Build history of the part. All positions in model axes, mm. Round coordinates to 2 decimals unless told otherwise and drop trailing zeros. One line per item, written item: value. Start each with the question number.
Item 1: Pin check, flat tip, straight feed: pin 1 (4 mm diameter, centred on x = 0, y = 0, fed in from +Z). Stop position of the tip, or through.
Item 2: Probe L1, parallel to X at y = 0, z = 8.5; L2, parallel to Y at x = -1, z = 9. List the from-to ranges inside material, lowest first.
Item 3: Two-plate mould, pull along X, no slides. Class faces 1 (the flat face through (11.5, 0, 11)), 2 (the flat face through (0, -11.5, 11)), 3 (the cylindrical face through (-0.195, 1.487, 11.579)): +X half, -X half, draft (parallel to the pull), parting line (faces both ways), or undercut.
```python
from build123d import *

# Parameters (mm, degrees)
SKETCH_W        = 23
SKETCH_H        = 23
PAD_DEPTH       = 23
SKETCH001_R     = 1.5
POCKET_DEPTH    = 23.001
CHAMFER_1_ANGLE = 60
CHAMFER_1_SIZE  = 2.75
CHAMFER_2_ANGLE = 60
CHAMFER_2_SIZE  = 2.75
FILLET_R        = 4


with BuildPart() as part:
    # Sketch → Pad (new body)
    with BuildSketch(Plane.XY):
        Rectangle(SKETCH_W, SKETCH_H)
    extrude(amount=PAD_DEPTH)

    # Sketch001 (on Face6 of Pad) → Pocket (cut, through all)
    with BuildSketch(Plane.XY.offset(23)):
        Circle(SKETCH001_R)
    extrude(amount=-POCKET_DEPTH, mode=Mode.SUBTRACT)

    # Chamfer 1
    chamfer_1_edges = [part.edges().sort_by_distance(p)[0] for p in [
        (-1.5, 0, 23),
    ]]
    chamfer_1_side = part.faces().sort_by_distance((-11.174731, 0, 23))[0]
    chamfer(chamfer_1_edges, length=CHAMFER_1_SIZE, angle=CHAMFER_1_ANGLE, reference=chamfer_1_side)

    # Chamfer 2
    chamfer_2_edges = [part.edges().sort_by_distance(p)[0] for p in [
        (-1.5, 0, 0),
    ]]
    chamfer_2_side = part.faces().sort_by_distance((-11.174731, 0, 0))[0]
    chamfer(chamfer_2_edges, length=CHAMFER_2_SIZE, angle=CHAMFER_2_ANGLE, reference=chamfer_2_side)

    # Fillet
    fillet_edges = [part.edges().sort_by_distance(p)[0] for p in [
        (-1.5, 0, 4.76314),
        (-1.5, 0, 18.23686),
    ]]
    fillet(fillet_edges, radius=FILLET_R)


solid = part.part
```
Output:
1. pin 1: stops at z = 19.1
2. L1: x = -11.5 to -1.5, 1.5 to 11.5
2. L2: y = -11.5 to -1.12, 1.12 to 11.5
3. face 1: +X half
3. face 2: draft
3. face 3: undercut
